from build123d import *

# Parameters (mm, degrees)
CUT_EXTRUDE1_START          = -6.35
CUT_EXTRUDE1_DEPTH          = 190.5
BOSS_EXTRUDE4_REACH         = 233.927
BOSS_EXTRUDE5_DEPTH         = 25.4
SKETCH3_W                   = 2.54
SKETCH3_H                   = 39.37
BOSS_EXTRUDE1_DEPTH         = 95.25
SKETCH11_R                  = 3.175
CUT_EXTRUDE6_DEPTH          = 251.563629798
SKETCH12_R                  = 1.524
CUT_EXTRUDE7_DEPTH          = 10.16
SKETCH5_W                   = 190.291482803
SKETCH5_H                   = 88.9
CUT_EXTRUDE2_DEPTH          = 3.81
SKETCH6_W                   = 182.671482803
SKETCH6_H                   = 81.28
CUT_EXTRUDE3_DEPTH          = 12.7
SKETCH14_W                  = 190.5
SKETCH14_H                  = 10.414
CUT_EXTRUDE8_DEPTH          = 179.366063356
SKETCH15_W                  = 139.7
SKETCH15_H                  = 5.08
BOSS_EXTRUDE6_DEPTH         = 12.7
F_1_4_0_25_DIAMETER_HOLE1_D = 6.35


with BuildPart() as part:
    # Sketch1 → Loft1 section 0
    with BuildSketch(Plane.XY):
        with BuildLine():
            Line((101.6, 0), (101.6, 12.7))
            Line((101.6, 12.7), (-101.6, 12.7))
            Line((-101.6, 12.7), (-101.6, 0))
            Line((-101.6, 0), (-95.25, 0))
            Line((-95.25, 0), (-95.25, 6.35))
            Line((-95.25, 6.35), (95.25, 6.35))
            Line((95.25, 6.35), (95.25, 0))
            Line((95.25, 0), (101.6, 0))
        make_face()
    # Sketch2 → Loft1 section 1
    with BuildSketch(Plane.XY.offset(-114.3)):
        with BuildLine():
            Line((-95.25, 0), (-95.25, 38.1))
            Line((-95.25, 38.1), (95.25, 38.1))
            Line((95.25, 38.1), (95.25, 0))
            Line((95.25, 0), (101.6, 0))
            Line((101.6, 0), (101.6, 44.45))
            Line((101.6, 44.45), (-101.6, 44.45))
            Line((-101.6, 44.45), (-101.6, 0))
            Line((-101.6, 0), (-95.25, 0))
        make_face()
    loft()

    # Sketch4 → Cut-Extrude1 (cut)
    with BuildSketch(Plane(origin=(101.6, 0, 0), x_dir=(0, 0, -1), z_dir=(1, 0, 0)).offset(CUT_EXTRUDE1_START)):
        Polygon((12.7, 32.737292081), (5.278114464, 32.737292081), (5.278114464, 14.166142907), (15.549865586, 5.547120329), (19.654278654, 10.392445124), (12.7, 16.227777778), align=None)
    extrude(amount=-CUT_EXTRUDE1_DEPTH, mode=Mode.SUBTRACT)

    # Sketch7 → Boss-Extrude4 (add, up to next)
    with BuildSketch(Plane.ZY.offset(-95.25), mode=Mode.PRIVATE) as boss_extrude4_sk1:
        Polygon((0, 6.35), (-2.44733549, 7.029815414), (-2.44733549, 5.08), (0, 5.08), align=None)
    boss_extrude4_tool1 = extrude(boss_extrude4_sk1.sketch, amount=BOSS_EXTRUDE4_REACH, mode=Mode.PRIVATE) - part.part
    add(boss_extrude4_tool1.solids().sort_by_distance((95.25, 5.896915, -1.309787))[0])

    # Sketch9 → Boss-Extrude5 (add)
    with BuildSketch(Plane(origin=(0, 0, -114.3), x_dir=(-1, 0, 0), z_dir=(0, 0, -1))):
        Polygon((-95.25, 0), (-101.6, 0), (-101.6, 44.45), (101.6, 44.45), (101.6, 0), (95.25, 0), (95.25, 38.1), (-95.25, 38.1), align=None)
    extrude(amount=BOSS_EXTRUDE5_DEPTH)

    # Sketch3 → Boss-Extrude1 (add, symmetric)
    with BuildSketch(Plane(origin=(0, 0, 0), x_dir=(0, 0, -1), z_dir=(1, 0, 0))):
        with Locations((138.43, 24.765)):
            Rectangle(SKETCH3_W, SKETCH3_H)
    extrude(amount=BOSS_EXTRUDE1_DEPTH, both=True)

    # Sketch11 → Cut-Extrude6 (cut, through all)
    with BuildSketch(Plane.ZY.offset(101.6)):
        with Locations((-129.032, 44.45)):
            Circle(SKETCH11_R)
    extrude(amount=-CUT_EXTRUDE6_DEPTH, mode=Mode.SUBTRACT)

    # Sketch12 → Cut-Extrude7 (cut)
    with BuildSketch(Plane(origin=(0, 44.45, 0), x_dir=(1, 0, 0), z_dir=(0, 1, 0))):
        with Locations(Location((98.425, 123.952, 0), (0, 0, 180))):
            Circle(SKETCH12_R)
        with Locations((98.425, 134.112)):
            Circle(SKETCH12_R)
        with Locations(Location((-98.425, 134.112, 0), (0, 0, 180))):
            Circle(SKETCH12_R)
        with Locations((-98.425, 123.952)):
            Circle(SKETCH12_R)
    extrude(amount=-CUT_EXTRUDE7_DEPTH, mode=Mode.SUBTRACT)

    # Sketch5 → Cut-Extrude2 (cut)
    with BuildSketch(Plane(origin=(0, 11.79025788, 3.275071633), x_dir=(1, 0, 0), z_dir=(0, 0.9635179096299408, 0.2676438637860946))):
        with Locations((-0.104258598, 74.316283438)):
            Rectangle(SKETCH5_W, SKETCH5_H)
    extrude(amount=-CUT_EXTRUDE2_DEPTH, mode=Mode.SUBTRACT)

    # Sketch6 → Cut-Extrude3 (cut)
    with BuildSketch(Plane(origin=(0, 8.119254644, 2.255348512), x_dir=(1, 0, 0), z_dir=(0, 0.9635179096299407, 0.26764386378609456))):
        with Locations((-0.104258599, 74.316283438)):
            Rectangle(SKETCH6_W, SKETCH6_H)
    extrude(amount=-CUT_EXTRUDE3_DEPTH, mode=Mode.SUBTRACT)

    # Sketch14 → Cut-Extrude8 (cut, through all)
    with BuildSketch(Plane(origin=(0, 44.45, 0), x_dir=(1, 0, 0), z_dir=(0, 1, 0))):
        with Locations((0, 129.032)):
            Rectangle(SKETCH14_W, SKETCH14_H)
    extrude(amount=-CUT_EXTRUDE8_DEPTH, mode=Mode.SUBTRACT)

    # Sketch15 → Boss-Extrude6 (add)
    with BuildSketch(Plane(origin=(101.6, 0, 0), x_dir=(0, 0, -1), z_dir=(1, 0, 0))):
        with Locations((69.85, 2.54)):
            Rectangle(SKETCH15_W, SKETCH15_H)
    boss_extrude6 = extrude(amount=BOSS_EXTRUDE6_DEPTH)

    # 1/4 (0.25) Diameter Hole1 (through all)
    with Locations(Plane(origin=(0, 5.08, 0), x_dir=(1, 0, 0), z_dir=(0, 1, 0))):
        with Locations((107.95, 16.757307422), (107.95, 131.057307422)):
            f_1_4_0_25_diameter_hole1 = Hole(F_1_4_0_25_DIAMETER_HOLE1_D / 2)

    # Mirror1: Boss-Extrude6 across plane
    add(boss_extrude6.mirror(Plane(origin=(0, 0, 0), x_dir=(0, 0, 1), z_dir=(1, 0, 0))))

    # Mirror2: 1/4 (0.25) Diameter Hole1 across plane
    add(f_1_4_0_25_diameter_hole1.mirror(Plane(origin=(0, 0, 0), x_dir=(0, 0, 1), z_dir=(1, 0, 0))), mode=Mode.SUBTRACT)


solid = part.part
For this review, take the finished solid that the model builds, in its own axes (mm). A direction names the side the tool comes from. Give positions to 0.01 mm unless a question says otherwise; leave off trailing zeros. Loops run counter-clockwise (first coordinate to the right, second up) from the corner with the lowest first, then second, coordinate; pieces in that order, holes last. Notation, with made-up numbers: (74, 29.25) - (119, 29.25) arc R24 cw to (119, 40.25) - close; hole circle Ø6 at (-8, 35). An arc over 180 degrees is marked (long way). Write each question's results on one line, items separated by ' | '.
(1) For line 1 along Z through (x, y) = (107.95, 2.1); line 2 along X through (y, z) = (26.5, -91); line 3 along Z through (x, y) = (24, 6), list the stretches that pass through material, from the lowest coordinate up.
Conclusion:
line 1: -139.7 to -134.23, -127.88 to -19.93, -13.58 to 0 | line 2: -101.6 to -95.25, 95.25 to 101.6 | line 3: -139.7 to -137.16, -2.45 to 0
(2) Take a section at C-C (x = 107.95). Give the boundary of the cut face in (y, z), then the cut area to 3 significant figures.
Conclusion:
outline: (0, -139.7) - (5.08, -139.7) - (5.08, -134.23) - (0, -134.23) - close; (0, -127.88) - (5.08, -127.88) - (5.08, -19.93) - (0, -19.93) - close; (0, -13.58) - (5.08, -13.58) - (5.08, 0) - (0, 0) - close | area: 645 mm^2
(3) Take a section at D-D (z = -117.5). Give the boundary of the cut face in (x, y), then the cut area to 3 significant figures.
Conclusion:
outline: (-114.3, 0) - (-95.25, 0) - (-95.25, 38.1) - (95.25, 38.1) - (95.25, 0) - (114.3, 0) - (114.3, 5.08) - (101.6, 5.08) - (101.6, 44.45) - (-101.6, 44.45) - (-101.6, 5.08) - (-114.3, 5.08) - close | area: 1,900 mm^2
(4) For pin 1 Ø2.5 at (x, z) = (-98.425, -123.952) entering from +Y; pin 2 Ø5 at (x, y) = (17.5, 18.5) entering from +Z; pin 3 Ø8 at (x, z) = (-14, -25) entering from +Y, all flat-tipped, find the tip position at first contact; note any pin that passes through.
Conclusion:
pin 1: y = 34.29 | pin 2: z = -12.7 | pin 3: y = 19.78
(5) Take a section at A-A (x = -30.5). State how many separate pieces and enclosed holes the cut face has, then the cut area to 3 significant figures.
Conclusion:
separate pieces: 4 | enclosed holes: 0 | area: 335 mm^2
(6) For faces 1 (the flat face through (-91.44, 27, -69)), 2 (the flat face through (1, 21, -137.16)), 3 (the flat face through (-101.6, 21, -84)), 4 (the flat face through (101.6, 20, -84)), list the 3-axis set-ups (+Z, -Z, +X, -X, +Y, -Y) from which the entire face can be reached by the end or side of a thin tool; tool diameter is ignored.
Conclusion:
face 1: +Y, -Y | face 2: -Y | face 3: +Z, -Z, -X, +Y | face 4: +Z, -Z, +X, +Y
(7) Draft analysis for pull direction Z (two halves, no side actions). For faces 5 (the flat face through (2, 8, 0)), 6 (the flat face through (-114.3, 3, -69)), 7 (the cylindrical face through (108.4, 2.5, -134.2)), state which applies: +Z half, -Z half, draft (parallel to the pull), parting line (faces both ways), or undercut.
Conclusion:
face 5: +Z half | face 6: draft | face 7: undercut
(8) Take a section at B-B (z = -66). Give the boundary of the cut face in (x, y), then the cut area to 3 significant figures.
Conclusion:
outline: (-114.3, 0) - (-95.25, 0) - (-95.25, 24.68) - (-91.44, 24.68) - (-91.44, 27.08) - (-95.25, 27.08) - (-95.25, 31.03) - (-101.6, 31.03) - (-101.6, 5.08) - (-114.3, 5.08) - close; (91.23, 24.68) - (95.25, 24.68) - (95.25, 0) - (114.3, 0) - (114.3, 5.08) - (101.6, 5.08) - (101.6, 31.03) - (95.04, 31.03) - (95.04, 27.08) - (91.23, 27.08) - close | area: 543 mm^2
